```python
from build123d import *

# Parameters (mm, degrees)
F3_D     = 5.1054
F3_DEPTH = 7.62
F3_TIP   = 1.5338169022


with BuildPart() as f1:
    # F0 (on Front) → F1 (revolve)
    with BuildSketch(Plane.XZ):
        with BuildLine():
            Line((19.05, 12.7), (0, 12.7))
            Line((0, 12.7), (0, 0))
            Line((0, 0), (19.05, 0))
            Line((19.05, 0), (19.05, 0.7874))
            Line((19.05, 0.7874), (16.2052, 0.7874))
            ThreePointArc((16.2052, 0.7874), (16.0255948776, 0.8617948776), (15.9512, 1.0414))
            Line((15.9512, 1.0414), (15.9512, 3.175))
            Line((15.9512, 3.175), (15.9512, 5.3086))
            ThreePointArc((15.9512, 5.3086), (16.0255948776, 5.4882051224), (16.2052, 5.5626))
            Line((16.2052, 5.5626), (19.05, 5.5626))
            Line((19.05, 5.5626), (19.05, 7.1374))
            Line((19.05, 7.1374), (16.2052, 7.1374))
            ThreePointArc((16.2052, 7.1374), (16.0255948776, 7.2117948776), (15.9512, 7.3914))
            Line((15.9512, 7.3914), (15.9512, 9.525))
            Line((15.9512, 9.525), (15.9512, 11.6586))
            ThreePointArc((15.9512, 11.6586), (16.0255948776, 11.8382051224), (16.2052, 11.9126))
            Line((16.2052, 11.9126), (19.05, 11.9126))
            Line((19.05, 11.9126), (19.05, 12.7))
        make_face()
    revolve(axis=Axis((0, 0, 6.35), (0, 0, -1)))

    # F3
    with Locations(Plane.XY.offset(12.7)):
        with Locations((0, 0)):
            Hole(F3_D / 2, depth=F3_DEPTH)
            with Locations((0, 0, -(F3_DEPTH + F3_TIP / 2))):  # 118° drill point
                Cone(0, F3_D / 2, F3_TIP, mode=Mode.SUBTRACT)


solid = f1.part
```
Input: part model. Units: mm. Frame: model coordinates. A direction names the side the tool comes from. Round coordinates to 2 decimals unless told otherwise and drop trailing zeros. Loops run counter-clockwise (first coordinate to the right, second up) from the corner with the lowest first, then second, coordinate; pieces in that order, holes last. Notation, with made-up numbers: (82, 83.25) -> (86, 83.25) arc R16 ccw to (86, 98.25) -> close; hole circle Ø7 at (-7.5, 55.25). An arc over 180 degrees is marked (long way). One line per item, written item: value.
(1) Pin query (flat end, axial travel): pin 1 (6 mm diameter, centred on y = -4, z = 11, fed in from -X); pin 2 (3 mm diameter, centred on x = -8.5, z = 11, fed in from +Y); pin 3 (2 mm diameter, centred on x = -12.5, z = 6, fed in from -Y). Return the tip coordinate at first contact, or that it passes through.
Geometry check:
pin 1: x = -19.02
pin 2: y = 17.59
pin 3: y = -15.19
(2) Material intervals for line 1 (Z direction, x = 14, y = 12.5); line 2 (Y direction, x = 0, z = 7); line 3 (X direction, y = 0, z = 10.5), sorted ascending. Write a range as [from, to].
Geometry check:
line 1: [0, 0.79], [5.56, 7.14], [11.91, 12.7]
line 2: [-19.05, -2.55], [2.55, 19.05]
line 3: [-15.95, -2.55], [2.55, 15.95]
(3) Mould query, pull axis Y, two halves, no side actions, for faces 3 (the face through (-10, -13, 0.787)), 4 (the face through (-15.12, 11.59, 0.4)), 5 (the face through (-2.435, 0.767, 8.837)), 6 (the face through (0.42, 0.13, 3.81)). Classes: pulls with the +Y half, pulls with the -Y half, needs draft (parallel to the pull), parting line crosses it, or undercut.
Geometry check:
face 3: needs draft
face 4: parting line crosses it
face 5: undercut
face 6: undercut
(4) Set-up query: faces 1 (the face through (-15.12, 11.59, 12.31)), 2 (the face through (10, -13, 5.563)). Return all of +Z, -Z, +X, -X, +Y, -Y with unobstructed straight access to the full face (end or side cutting, diameter ignored); none if empty.
Geometry check:
face 1: +Z, -Z
face 2: none
(5) Section A-A (z = 9). Return the cut outline in (x, y), plus the area to 3 significant figures.
Geometry check:
outline: circle Ø31.9 at (0, 0); hole circle Ø5.11 at (0, 0)
area: 779 mm2
